from build123d import *

# Parameters (mm, degrees)
SKETCH_R     = 2.5
PAD_DEPTH    = 2
CHAMFER_SIZE = 0.35


with BuildPart() as part:
    # Sketch → Pad (new body, symmetric)
    with BuildSketch(Plane.XY):
        Polygon((0, -4.618802), (4, -2.309401), (4, 2.309401), (0, 4.618802), (-4, 2.309401), (-4, -2.309401), align=None)
        Circle(SKETCH_R, mode=Mode.SUBTRACT)
    extrude(amount=PAD_DEPTH, both=True)

    # Sketch001 → Groove (revolve, cut)
    with BuildSketch(Plane.YZ):
        Polygon((-4, 2), (-4.618802, 1.642734), (-4.618802, 2), align=None)
        Polygon((-4, -2), (-4.618802, -2), (-4.618802, -1.642734), align=None)
    revolve(axis=Axis((0, 0, 0), (0, 0, 1)), mode=Mode.SUBTRACT)

    # Chamfer
    chamfer_edges = [part.edges().sort_by_distance(p)[0] for p in [
        (-2.5, 0, 2),
        (-2.5, 0, -2),
    ]]
    chamfer(chamfer_edges, length=CHAMFER_SIZE)


solid = part.part
Verification items for the finished model (mm, model axes). Round coordinates to 2 decimals unless told otherwise and drop trailing zeros. Order: outer loops, then holes, each group sorted by start corner. A loop starts at its lowest first (then second) coordinate and runs counter-clockwise, first axis right, second up.
1. Section check A-A on z = -1.25. Record the cut outline in (x, y), then the cut area to 3 significant figures.
Final values:
outline: (-4, -2.31) - (0, -4.62) - (4, -2.31) - (4, 2.31) - (0, 4.62) - (-4, 2.31) - close; hole circle Ø5 at (0, 0)
area: 35.8 mm2
2. Thickness scan on L1, parallel to X at y = 1.5, z = 0.2; L2, parallel to Y at x = 2.25, z = -1.7; L3, parallel to Y at x = -1.75, z = -1.45. Record the ranges inside material, lowest first.
Final values:
L1: x = -4 to -2, 2 to 4
L2: y = -3.32 to -1.2, 1.2 to 3.32
L3: y = -3.61 to -1.79, 1.79 to 3.61
3. Go/stop test with flat-tipped pins: P1, Ø1.5, axis at x = 2.5, z = -1.5, coming from the -Y side; P2, Ø2, axis at x = 2.5, z = -0.5, coming from the -Y side. Record where each tip stops, or that it passes through.
Final values:
P1: stops at y = -3.61
P2: stops at y = -3.75
4. Release check for a two-part mould opening along Y. For faces 1 (the conical face through (3.589, -2.084, 1.913)), 2 (the cylindrical face through (-0.54, -2.44, -0.02)), 3 (the conical face through (0.01, 4.148, -1.915)) record: +Y half, -Y half, draft (parallel to the pull), parting line (faces both ways), or undercut.
Final values:
face 1: -Y half
face 2: undercut
face 3: +Y half
